Here's how the part is built. I have some questions about the finished solid (model axes, mm). A direction names the side the tool comes from. Give positions to 0.01 mm unless a question says otherwise; leave off trailing zeros. Write each loop counter-clockwise with the first axis right and the second up, starting at its lowest first coordinate (ties: lowest second). Pieces come first, ordered by that corner, then holes. Notation, with made-up numbers: (88.5, 86.25) - (122.5, 86.25) arc R16 cw to (122.5, 93.25) - close; hole circle Ø7 at (-31, 11). An arc over 180 degrees is marked (long way). One line per item, written item: value. Start each with the question number.
1) Imagine slicing it at C-C on z = 114.2. Count the separate pieces of the cut face and the enclosed holes in it, plus the area to 3 significant figures.
2) Imagine slicing it at D-D on z = 150.5. Write out the boundary of the cut face in (x, y), plus the area to 3 significant figures.
3) Imagine slicing it at A-A on x = -11. Write out the boundary of the cut face in (y, z).
4) Imagine slicing it at B-B on y = -14. Write out the boundary of the cut face in (x, z), plus the area to 3 significant figures.
5) Please list where these lines run through material, in increasing order: L1, parallel to Y at x = 134.5, z = 114; L2, parallel to X at y = -222, z = 136.5; L3, parallel to Y at x = 209, z = 114. Write a range as [from, to].
6) On a 3-axis mill with a long thin cutter (end or side, diameter ignored), from which of +Z, -Z, +X, -X, +Y, -Y can I reach the whole of each face in a straight line? I mean faces 3 (the flat face through (78, -268.642, 80)), 4 (the flat face through (78, -267.642, 80)). Say none if no direction works.
7) We'd pull the mould along Z, two halves only. Please class faces 1 (the cylindrical face through (-57.233, 90.063, 101.997)), 2 (the flat face through (193.75, 177.57, 79.87)): +Z half, -Z half, draft (parallel to the pull), parting line (faces both ways), or undercut.
from build123d import *

# Parameters (mm, degrees)
BOSS_EXTRUDE1_DEPTH = 162
SKETCH2_R           = 12.5
CUT_EXTRUDE1_DEPTH  = 413.402232553


with BuildPart() as part:
    # Sketch1 → Boss-Extrude1 (new body)
    with BuildSketch(Plane.XY):
        Polygon((-57.739503943, 162.772609534), (-27.153717505, 193.358395972), (179.374709619, 193.358395972), (209.960496057, 162.772609534), (209.960496057, -238.055817591), (179.374709619, -268.641604028), (-27.153717505, -268.641604028), (-57.739503943, -238.055817591), align=None)
        Polygon((-56.739503943, 162.358395972), (-26.739503943, 192.358395972), (178.960496057, 192.358395972), (208.960496057, 162.358395972), (208.960496057, -237.641604028), (178.960496057, -267.641604028), (-26.739503943, -267.641604028), (-56.739503943, -237.641604028), align=None, mode=Mode.SUBTRACT)
    extrude(amount=BOSS_EXTRUDE1_DEPTH)

    # Sketch2 → Cut-Extrude1 (cut, through all)
    with BuildSketch(Plane(origin=(209.960496057, 0, 0), x_dir=(0, 0, -1), z_dir=(1, 0, 0))):
        with Locations(Location((-114.2, -168.055817591, 0), (0, 0, 90))):
            Circle(SKETCH2_R)
        with Locations(Location((-114.2, 92.772609534, 0), (0, 0, 90))):
            Circle(SKETCH2_R)
    extrude(amount=-CUT_EXTRUDE1_DEPTH, mode=Mode.SUBTRACT)


solid = part.part
Numbers:
1. separate pieces: 4
1. enclosed holes: 0
1. area: 1,280 mm^2
2. outline: (-57.74, -238.06) - (-27.15, -268.64) - (179.37, -268.64) - (209.96, -238.06) - (209.96, 162.77) - (179.37, 193.36) - (-27.15, 193.36) - (-57.74, 162.77) - close; hole (-56.74, -237.64) - (-26.74, -267.64) - (178.96, -267.64) - (208.96, -237.64) - (208.96, 162.36) - (178.96, 192.36) - (-26.74, 192.36) - (-56.74, 162.36) - close
2. area: 1,380 mm^2
3. outline: (-268.64, 0) - (-267.64, 0) - (-267.64, 162) - (-268.64, 162) - close; (192.36, 0) - (193.36, 0) - (193.36, 162) - (192.36, 162) - close
4. outline: (-57.74, 0) - (-56.74, 0) - (-56.74, 162) - (-57.74, 162) - close; (208.96, 0) - (209.96, 0) - (209.96, 162) - (208.96, 162) - close
4. area: 324 mm^2
5. L1: [-268.64, -267.64], [192.36, 193.36]
5. L2: [-57.74, -56.74], [208.96, 209.96]
5. L3: [-239.02, -180.55], [-155.56, 80.27], [105.27, 163.73]
6. face 3: +Z, -Z, +X, -X, -Y
6. face 4: +Z, -Z
7. face 1: undercut
7. face 2: draft
